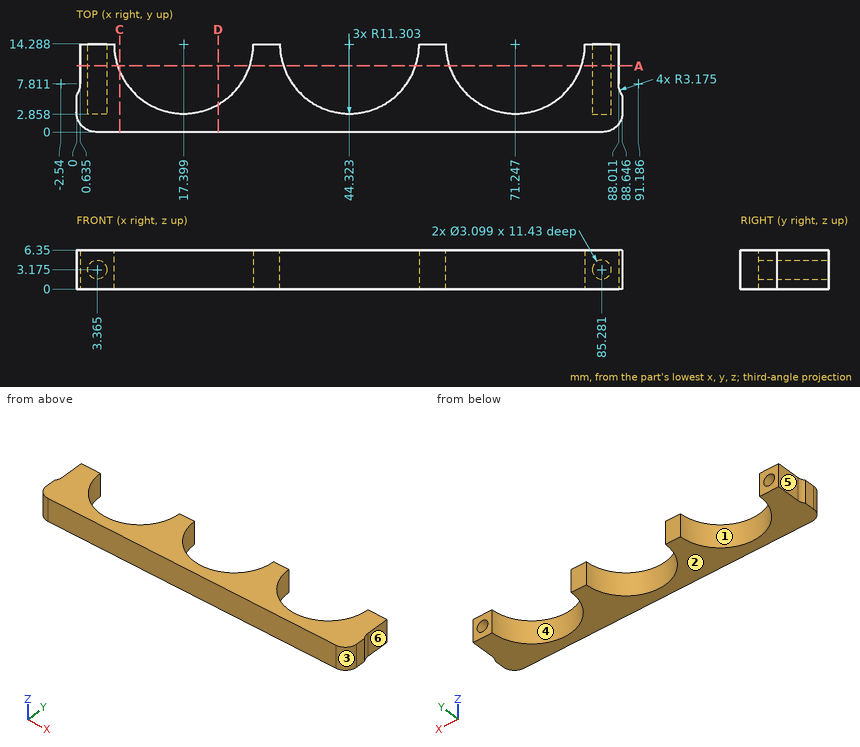
Part print with two shaded views. Sizes in mm from the minimum x, y, z corner. A direction names the side the tool comes from. Round coordinates to 2 decimals unless told otherwise and drop trailing zeros. Loops run counter-clockwise (first coordinate to the right, second up) from the corner with the lowest first, then second, coordinate; pieces in that order, holes last. Notation, with made-up numbers: M 85.25,26.25 L 143.25,26.25 A32 ccw 143.25,57.25 Z; hole C 77,60 d8. An arc over 180 degrees is marked long. Return JSON: item names as keys, results as strings. Group by question number.
(1) Drop a flat-ended pin along its axis: P1, Ø1, axis at y = 9, z = 1.5, coming from the +X side. Give the stop position or say it passes through.
(2) Saw through at D-D, the plane x = 23. List the corners of the cut face in (y, z), and give its area (3 significant figures).
(3) Wall check: probe 1 along X at (y, z) = (9, 4) (1 decimal); probe 2 along X at (y, z) = (9.5, 5) (1 decimal); probe 3 along X at (y, z) = (7, 1.25) (1 decimal). Give the ranges that are in metal, low to high. Write a range as [from, to].
(4) Saw through at A-A, the plane y = 10.75. Give the number of separate pieces and of enclosed holes in the cut face, and give its area (3 significant figures).
(5) Mould opens along X. For the marked faces 1, 2 and 3 say: +X half, -X half, draft (parallel to the pull), parting line (faces both ways), or undercut.
(6) Saw through at C-C, the plane x = 7. List the corners of the cut face in (y, z).
(7) Tool access for the marked faces 4, 5 and 6: list every direction of +Z, -Z, +X, -X, +Y, -Y with a clear straight run to the whole face (end or side of a thin tool).
Answer list:
{
 "1": {"P1": "x = 88.01"},
 "2": {"outline": "M 0,0 L 4.47,0 L 4.47,6.35 L 0,6.35 Z", "area": "28.4 mm2"},
 "3": {"probe 1": "[0.6, 2.1], [4.7, 7.4], [27.4, 34.3], [54.3, 61.3], [81.2, 84], [86.6, 88]", "probe 2": "[0.6, 7.2], [27.6, 34.1], [54.6, 61], [81.5, 88]", "probe 3": "[0.5, 8.8], [26, 35.7], [53, 62.6], [79.9, 88.1]"},
 "4": {"separate pieces": "4", "enclosed holes": "2", "area": "131 mm2"},
 "5": {"face 1": "undercut", "face 2": "draft", "face 3": "+X half"},
 "6": {"outline": "M 0,0 L 9.86,0 L 9.86,6.35 L 0,6.35 Z"},
 "7": {"face 4": "+Z, -Z, +Y", "face 5": "+Z, -Z, -X, +Y", "face 6": "+Z, -Z, +X, +Y"}
}
